from build123d import *

# Parameters (mm, degrees)
SKETCH1_W           = 139.7
SKETCH1_H           = 152.4
BOSS_EXTRUDE1_DEPTH = 6.35
FILLET1_R           = 12.7
SKETCH2_W           = 101.6
SKETCH2_H           = 25.4
BOSS_EXTRUDE2_DEPTH = 6.35
FILLET2_R           = 1.27


with BuildPart() as part:
    # Sketch1 → Boss-Extrude1 (new body)
    with BuildSketch(Plane(origin=(0, 0, 0), x_dir=(1, 0, 0), z_dir=(0, 1, 0))):
        Rectangle(SKETCH1_W, SKETCH1_H)
        with BuildLine():
            ThreePointArc((54.864, -50.8), (53.673681959, -53.673681959), (50.8, -54.864))
            Line((50.8, -54.864), (-50.8, -54.864))
            ThreePointArc((-50.8, -54.864), (-54.864, -50.8), (-50.8, -46.736))
            Line((-50.8, -46.736), (50.8, -46.736))
            ThreePointArc((50.8, -46.736), (53.673681959, -47.926318041), (54.864, -50.8))
        make_face(mode=Mode.SUBTRACT)
        with BuildLine():
            ThreePointArc((-50.8, 46.736), (-54.864, 50.8), (-50.8, 54.864))
            Line((-50.8, 54.864), (50.8, 54.864))
            ThreePointArc((50.8, 54.864), (53.673681959, 53.673681959), (54.864, 50.8))
            ThreePointArc((54.864, 50.8), (53.673681959, 47.926318041), (50.8, 46.736))
            Line((50.8, 46.736), (-50.8, 46.736))
        make_face(mode=Mode.SUBTRACT)
    extrude(amount=BOSS_EXTRUDE1_DEPTH)

    # Fillet1
    fillet1_edges = [part.edges().sort_by_distance(p)[0] for p in [
        (-69.85, 3.175, 76.2),
        (-69.85, 3.175, -76.2),
    ]]
    fillet(fillet1_edges, radius=FILLET1_R)

    # Sketch2 → Boss-Extrude2 (add)
    with BuildSketch(Plane(origin=(0, 6.35, 0), x_dir=(1, 0, 0), z_dir=(0, 1, 0))):
        with Locations((-120.65, 0)):
            Rectangle(SKETCH2_W, SKETCH2_H)
    extrude(amount=-BOSS_EXTRUDE2_DEPTH)

    # Fillet2
    fillet2_edges = [part.edges().sort_by_distance(p)[0] for p in [
        (69.85, 3.175, -76.2),
        (69.85, 3.175, 76.2),
        (-171.45, 3.175, 12.7),
        (-171.45, 3.175, -12.7),
    ]]
    fillet(fillet2_edges, radius=FILLET2_R)


solid = part.part
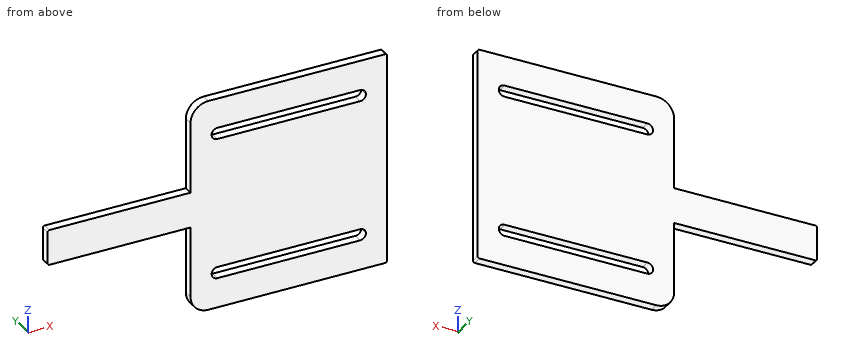
Read the model definition and answer for the solid it produces. Units are mm, in the model's axes. Round coordinates to 2 decimals unless told otherwise and drop trailing zeros. Write each loop counter-clockwise with the first axis right and the second up, starting at its lowest first coordinate (ties: lowest second). Pieces come first, ordered by that corner, then holes.
Q1. Find section B-B on x = -20.5. Determine the outline of the cut face in (y, z), and give its area (3 significant figures).
Values:
outline: (0, -76.2) - (6.35, -76.2) - (6.35, -54.86) - (0, -54.86) - close; (0, -46.74) - (6.35, -46.74) - (6.35, 46.74) - (0, 46.74) - close; (0, 54.86) - (6.35, 54.86) - (6.35, 76.2) - (0, 76.2) - close
area: 865 mm2
Q2. Straight lines are drawn through the part: line 1 (Z direction, x = -5.5, y = 2.75); line 2 (X direction, y = 5.75, z = 50.5); line 3 (Z direction, x = -104, y = 2). For each, find the intervals that lie inside material, in ascending order.
Values:
line 1: z = -76.2 to -54.86, -46.74 to 46.74, 54.86 to 76.2
line 2: x = -69.85 to -54.85, 54.85 to 69.85
line 3: z = -12.7 to 12.7
Q3. Find section D-D on z = -35. Determine the outline of the cut face in (x, y), and give its area (3 significant figures).
Values:
outline: (-69.85, 0) - (69.85, 0) - (69.85, 6.35) - (-69.85, 6.35) - close
area: 887 mm2
Q4. Find section C-C on x = -85.5. Determine the outline of the cut face in (y, z).
Values:
outline: (0, -12.7) - (6.35, -12.7) - (6.35, 12.7) - (0, 12.7) - close
Q5. Flat-ended cylindrical pins translate along their axes: P1, Ø3, axis at y = 4.5, z = -42.5, coming from the -X side; P2, Ø3, axis at x = -123, y = 4.5, coming from the -Z side. Find the tip coordinate at first contact, or state that the pin passes through.
Values:
P1: stops at x = -69.85
P2: stops at z = -12.7
Q6. Find section A-A on y = 4. Determine the outline of the cut face in (x, z), and give its area (3 significant figures).
Values:
outline: (-171.45, -11.43) arc R1.27 ccw to (-170.18, -12.7) - (-69.85, -12.7) - (-69.85, -63.5) arc R12.7 ccw to (-57.15, -76.2) - (68.58, -76.2) arc R1.27 ccw to (69.85, -74.93) - (69.85, 74.93) arc R1.27 ccw to (68.58, 76.2) - (-57.15, 76.2) arc R12.7 ccw to (-69.85, 63.5) - (-69.85, 12.7) - (-170.18, 12.7) arc R1.27 ccw to (-171.45, 11.43) - close; hole (-50.8, -54.86) - (50.8, -54.86) arc R4.06 ccw to (50.8, -46.74) - (-50.8, -46.74) arc R4.06 ccw to start; hole (-50.8, 46.74) - (50.8, 46.74) arc R4.06 ccw to (50.8, 54.86) - (-50.8, 54.86) arc R4.06 ccw to start
area: 22,000 mm2
